CAD build for the part. Positions are in the model's coordinates, mm. Face numbers are marked on the shaded views. A direction names the side the tool comes from. Give positions to 0.01 mm unless a question says otherwise; leave off trailing zeros. Write each loop counter-clockwise with the first axis right and the second up, starting at its lowest first coordinate (ties: lowest second). Pieces come first, ordered by that corner, then holes. Notation, with made-up numbers: (-14.75, 84) - (-5.75, 84) arc R29 cw to (-5.75, 105) - close; hole circle Ø6 at (60, -12). An arc over 180 degrees is marked (long way). Answer as a JSON object with one key per item and string values.
from build123d import *

# Parameters (mm, degrees)
BOSS_EXTRUDE1_DEPTH = 1.5
BOSS_EXTRUDE2_START = 2.3
SKETCH2_R           = 3.5
SKETCH2_R_2         = 2.4
BOSS_EXTRUDE2_DEPTH = 2.3
SKETCH3_R           = 1
CUT_EXTRUDE2_DEPTH  = 17.813387523


with BuildPart() as part:
    # Sketch1 → Boss-Extrude1 (new body)
    with BuildSketch(Plane(origin=(0, 0, 0), x_dir=(1, 0, 0), z_dir=(0, 1, 0))):
        with BuildLine():
            Line((0, 3.5), (14, 2))
            ThreePointArc((14, 2), (16, 0), (14, -2))
            Line((14, -2), (0, -3.5))
            ThreePointArc((0, -3.5), (-3.5, 0), (0, 3.5))
        make_face()
    extrude(amount=BOSS_EXTRUDE1_DEPTH)

    # Sketch2 → Boss-Extrude2 (add)
    with BuildSketch(Plane.XZ.offset(BOSS_EXTRUDE2_START)):
        with Locations(Location((0, 0, 0), (0, 0, 270))):
            Circle(SKETCH2_R)
        with Locations(Location((0, 0, 0), (0, 0, 270))):
            Circle(SKETCH2_R_2, mode=Mode.SUBTRACT)
    extrude(amount=-BOSS_EXTRUDE2_DEPTH)

    # Sketch3 → Cut-Extrude2 (cut, through all)
    with BuildSketch(Plane(origin=(0, 1.5, 0), x_dir=(1, 0, 0), z_dir=(0, 1, 0))):
        with Locations(Location((14, 0, 0), (0, 0, 270))):
            Circle(SKETCH3_R)
        with Locations(Location((11, 0, 0), (0, 0, 270))):
            Circle(SKETCH3_R)
        with Locations(Location((8, 0, 0), (0, 0, 270))):
            Circle(SKETCH3_R)
        with Locations(Location((5, 0, 0), (0, 0, 270))):
            Circle(SKETCH3_R)
    extrude(amount=-CUT_EXTRUDE2_DEPTH, mode=Mode.SUBTRACT)


solid = part.part
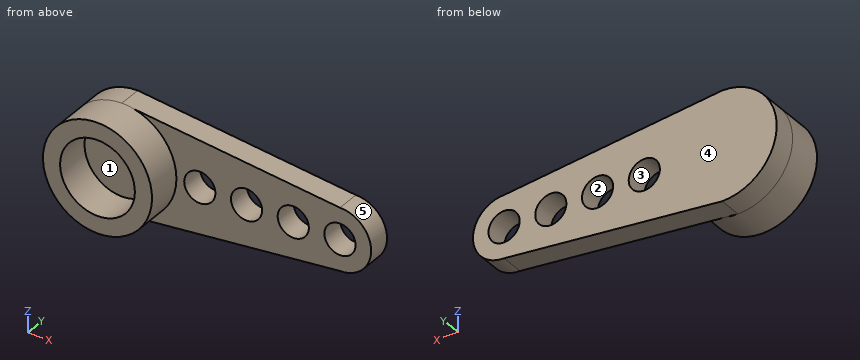
Item 1: Cut at D-D (y = -0.7). Give the cut face in (x, z), and give its area (3 significant figures).
Entries:
{"outline": "circle Ø7 at (0, 0); hole circle Ø4.8 at (0, 0)", "area": "20.4 mm2"}
Item 2: Cut at A-A (z = 0). Give the cut face in (x, y).
Entries:
{"outline": "(-3.5, -2.3) - (-2.4, -2.3) - (-2.4, 0) - (2.4, 0) - (2.4, -2.3) - (3.5, -2.3) - (3.5, 0) - (4, 0) - (4, 1.5) - (-3.5, 1.5) - close; (6, 0) - (7, 0) - (7, 1.5) - (6, 1.5) - close; (9, 0) - (10, 0) - (10, 1.5) - (9, 1.5) - close; (12, 0) - (13, 0) - (13, 1.5) - (12, 1.5) - close; (15, 0) - (16, 0) - (16, 1.5) - (15, 1.5) - close"}
Item 3: Cut at C-C (x = 11). Give the cut face in (y, z).
Entries:
{"outline": "(0, -2.32) - (1.5, -2.32) - (1.5, -1) - (0, -1) - close; (0, 1) - (1.5, 1) - (1.5, 2.32) - (0, 2.32) - close"}
Item 4: Which spindle directions (+Z, -Z, +X, -X, +Y, -Y) get a long thin tool onto all of the face, cutting with end or side? Do the marked faces 1 and 2. Say none if no direction does.
Entries:
{"face 1": "-Y", "face 2": "+Y, -Y"}
Item 5: Probe line 1 (X direction, y = 1, z = 0); line 2 (X direction, y = -1.8, z = 0); line 3 (Y direction, x = 3.75, z = -1). List the from-to ranges inside material, lowest first. Write a range as from..to.
Entries:
{"line 1": "-3.5..4, 6..7, 9..10, 12..13, 15..16", "line 2": "-3.5..-2.4, 2.4..3.5", "line 3": "0..1.5"}
Item 6: Mould opens along Z. For the marked faces 3, 4 and 5 say: +Z half, -Z half, draft (parallel to the pull), parting line (faces both ways), or undercut.
Entries:
{"face 3": "undercut", "face 4": "draft", "face 5": "parting line"}
Item 7: Cut at B-B (y = 0.8). Give the cut face in (x, z), and give its area (3 significant figures).
Entries:
{"outline": "(0, -3.5) - (14, -2) arc R2 ccw to (14, 2) - (0, 3.5) arc R3.5 ccw to start; hole circle Ø2 at (5, 0); hole circle Ø2 at (8, 0); hole circle Ø2 at (11, 0); hole circle Ø2 at (14, 0)", "area": "90.0 mm2"}
Item 8: Flat gauge pins, fed straight in: P1, Ø2, axis at y = 0, z = 1.5, coming from the +X side; P2, Ø2.5, axis at x = 8, z = 0, coming from the -Y side. Where does each tip first touch, or does it go through?
Entries:
{"P1": "x = 15.94", "P2": "y = 0"}
